Geometry: final body of the model. Coordinates: model frame, mm. A direction names the side the tool comes from. Give positions to 0.01 mm unless a question says otherwise; leave off trailing zeros. Write each loop counter-clockwise with the first axis right and the second up, starting at its lowest first coordinate (ties: lowest second). Pieces come first, ordered by that corner, then holes. Notation, with made-up numbers: (-6, -32) -> (46, -32) arc R29 cw to (46, 3) -> close; hole circle Ø9 at (53, 5). An arc over 180 degrees is marked (long way). Answer in a Markdown table with one row per item. Add a question column.
Item 1: First-contact query: P1, Ø4.5, axis at y = 13, z = -30.5, coming from the +X side; P2, Ø1.6, axis at y = 12.7, z = -30, coming from the +X side; P3, Ø3, axis at y = 12.5, z = 28, coming from the +X side. Flat tips, straight axial feed; report the tip coordinate or a pass-through.
Item 2: Section query A-A on y = 6.5. Output: boundary loops of the cut face in (x, z).
Item 3: Material intervals for probe 1 along Z at (x, y) = (33.25, 12.7); probe 2 along Y at (x, z) = (43, -30); probe 3 along Z at (x, y) = (-28, 6.25), sorted ascending. Write a range as from..to.
Item 4: Draft query along Y for faces 1 (the flat face through (-20, 13, 12.7)), 2 (the flat face through (-1, 25.4, -1)), 3 (the flat face through (49.187, 14, -30)), 4 (the flat face through (-1, 0, -1)). Return one class per face: +Y half, -Y half, draft (parallel to the pull), parting line (faces both ways), or undercut.
Item 5: Section query B-B on x = -18. Output: boundary loops of the cut face in (y, z).
Item 6: Access query for faces 5 (the flat face through (-50, 13, 1)), 6 (the flat face through (-20, 13, -12.7)), 7 (the flat face through (49.187, 14, 29)). Directions: +Z, -Z, +X, -X, +Y, -Y. A direction counts if a zero-diameter tool reaches every point of the face in a straight line with its end or side. Return the directions, or none.
```python
from build123d import *

# Parameters (mm, degrees)
SKETCH1_W                                   = 100
SKETCH1_H                                   = 160
SKETCH1_W_2                                 = 25.4
SKETCH1_H_2                                 = 25.4
BOSS_EXTRUDE1_DEPTH                         = 25.4
CBORE_FOR_0_BINDING_HEAD_MACHINE_SC_2_COUNT = 2
CBORE_FOR_0_BINDING_HEAD_MACHINE_SC_2_PITCH = 58.4


with BuildPart() as part:
    # Sketch1 → Boss-Extrude1 (new body)
    with BuildSketch(Plane(origin=(0, 0, 0), x_dir=(1, 0, 0), z_dir=(0, 1, 0))):
        Rectangle(SKETCH1_W, SKETCH1_H)
        with Locations((-19.49, 0)):
            Rectangle(SKETCH1_W_2, SKETCH1_H_2, mode=Mode.SUBTRACT)
    extrude(amount=BOSS_EXTRUDE1_DEPTH)

    # Sketch3 → CBORE for #0 Binding Head Machine Screw1 (revolve, cut)
    with BuildSketch(Plane(origin=(50, 12.7, 28.4), x_dir=(0, 0, -1), z_dir=(0, 1, 0))):
        Polygon((0, 0), (0, 30.53416509), (0.889, 30), (0.889, 0.8128), (1.98501, 0.8128), (1.98501, 0.87249), (2.8575, 0), align=None)
    cbore_for_0_binding_head_machine_screw1 = revolve(axis=Axis((56.35, 12.7, 28.4), (-1, 0, 0)), mode=Mode.SUBTRACT)

    # CBORE for _0 Binding Head Machine Sc 2: CBORE for #0 Binding Head Machine Screw1 ×2
    with Locations(*[(0, 0, -i * CBORE_FOR_0_BINDING_HEAD_MACHINE_SC_2_PITCH) for i in range(1, CBORE_FOR_0_BINDING_HEAD_MACHINE_SC_2_COUNT)]):
        add(cbore_for_0_binding_head_machine_screw1, mode=Mode.SUBTRACT)


solid = part.part
```
Findings below:
| question | item | result |
|---|---|---|
| 1 | P1 | stops at x = 49.98 |
| 1 | P2 | stops at x = 19.95 |
| 1 | P3 | stops at x = 49.19 |
| 2 | outline | (-50, -80) -> (50, -80) -> (50, 80) -> (-50, 80) -> close; hole (-32.19, -12.7) -> (-6.79, -12.7) -> (-6.79, 12.7) -> (-32.19, 12.7) -> close |
| 3 | probe 1 | z = -80..-30.89, -29.11..27.51, 29.29..80 |
| 3 | probe 2 | y = 0..11.81, 13.59..25.4 |
| 3 | probe 3 | z = -80..-12.7, 12.7..80 |
| 4 | face 1 | draft |
| 4 | face 2 | +Y half |
| 4 | face 3 | undercut |
| 4 | face 4 | -Y half |
| 5 | outline | (0, -80) -> (25.4, -80) -> (25.4, -12.7) -> (0, -12.7) -> close; (0, 12.7) -> (25.4, 12.7) -> (25.4, 80) -> (0, 80) -> close |
| 6 | face 5 | +Z, -Z, -X, +Y, -Y |
| 6 | face 6 | +Y, -Y |
| 6 | face 7 | +X |
